For this review, take the finished solid that the model builds, in its own axes (mm). Face numbers are marked on the shaded views. A direction names the side the tool comes from. Coordinates: 2 decimals unless noted, no trailing zeros. Loops run counter-clockwise (first coordinate to the right, second up) from the corner with the lowest first, then second, coordinate; pieces in that order, holes last. Notation, with made-up numbers: (70, 89.5) - (82, 89.5) arc R9 ccw to (82, 105.5) - close; hole circle Ø1 at (53, -11.75). An arc over 180 degrees is marked (long way). One line per item, written item: value. Start each with the question number.
1. To check wall thickness, follow line 1 (X direction, y = -2.5, z = 9.75); line 2 (X direction, y = 2.75, z = 9.75); line 3 (Z direction, x = 62, y = 3.5). State the ranges of each line that lie inside material, in increasing order. Write a range as from..to.
2. Take a section at A-A, the plane z = 5.5. State the section outline as (x, y) points, and give its area (3 significant figures).
3. Insertion check: pin 1 (1 mm diameter, centred on y = -2.5, z = 2.5, fed in from -X); pin 2 (1.6 mm diameter, centred on x = 98, y = 1, fed in from -Z); pin 3 (1 mm diameter, centred on y = -3, z = 10.5, fed in from -X). Each pin has a flat end and moves straight along its axis. Give the tip position at first contact, or say it passes through.
4. For the marked faces 3 and 4, list the 3-axis set-ups (+Z, -Z, +X, -X, +Y, -Y) from which the entire face can be reached by the end or side of a thin tool; tool diameter is ignored.
5. The part is to be moulded in two halves that separate along X. For the marked faces 1 and 2, say which applies: released by +X, released by -X, zero draft, split by the parting line, or undercut.
6. Take a section at B-B, the plane x = 43.5. State the section outline as (y, z) points.
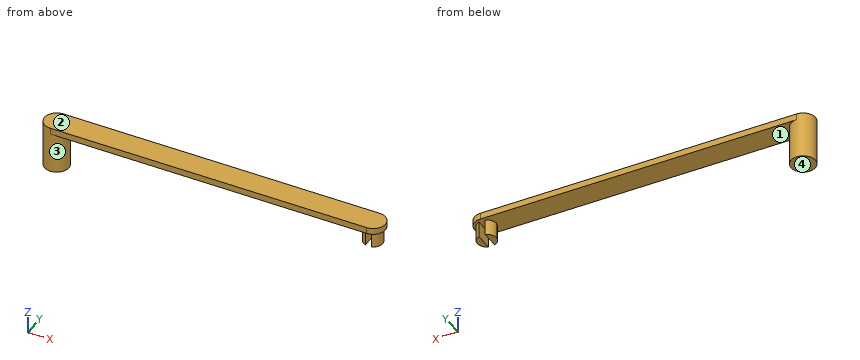
```python
from build123d import *

# Parameters (mm, degrees)
SKETCH1_R           = 3.85
BOSS_EXTRUDE1_DEPTH = 12.83
SKETCH2_R           = 3.85
BOSS_EXTRUDE3_DEPTH = 2
BOSS_EXTRUDE5_DEPTH = 5


with BuildPart() as part:
    # Sketch1 → Boss-Extrude1 (new body)
    with BuildSketch(Plane.XY):
        with Locations(Location((0, 0, 0), (0, 0, 180))):
            Circle(SKETCH1_R)
    extrude(amount=BOSS_EXTRUDE1_DEPTH)

    # Sketch2 → Boss-Extrude3 (add)
    with BuildSketch(Plane.XY.offset(12.83)):
        with Locations((100, 0)):
            Circle(SKETCH2_R)
        with BuildLine():
            Line((100, 3.85), (0, 3.85))
            ThreePointArc((0, 3.85), (2.722361108, 2.722361108), (3.85, 0))
            ThreePointArc((3.85, 0), (2.722361108, -2.722361108), (0, -3.85))
            Line((0, -3.85), (100, -3.85))
            ThreePointArc((100, -3.85), (96.15, 0), (100, 3.85))
        make_face()
        with BuildLine():
            ThreePointArc((3.85, 0), (2.722361108, 2.722361108), (0, 3.85))
            Line((0, 3.85), (0, -3.85))
            ThreePointArc((0, -3.85), (2.722361108, -2.722361108), (3.85, 0))
        make_face()
        with BuildLine():
            Line((0, -3.85), (0, 3.85))
            ThreePointArc((0, 3.85), (-3.85, 0), (0, -3.85))
        make_face()
    extrude(amount=BOSS_EXTRUDE3_DEPTH)

    # Sketch3 → Boss-Extrude5 (add)
    with BuildSketch(Plane(origin=(0, 0, 12.83), x_dir=(-1, 0, 0), z_dir=(0, 0, -1))):
        with BuildLine():
            Line((-101, -2.828427125), (-101, 2.828427125))
            ThreePointArc((-101, 2.828427125), (-103, 0), (-101, -2.828427125))
        make_face()
        with BuildLine():
            ThreePointArc((-97, 0), (-97.550510257, 1.732050808), (-99, 2.828427125))
            Line((-99, 2.828427125), (-99, -2.828427125))
            ThreePointArc((-99, -2.828427125), (-97.550510257, -1.732050808), (-97, 0))
        make_face()
    extrude(amount=BOSS_EXTRUDE5_DEPTH)


solid = part.part
```
Solutions:
1. line 1: -2.93..2.93, 98.34..99, 101..101.66
1. line 2: -2.69..2.69, 98.8..99, 101..101.2
1. line 3: 12.83..14.83
2. outline: circle Ø7.7 at (0, 0)
2. area: 46.6 mm2
3. pin 1: x = -3.29
3. pin 2: z = 7.83
3. pin 3: x = -2.93
4. face 3: -Z
4. face 4: -Z, +X, -X, +Y, -Y
5. face 1: undercut
5. face 2: zero draft
6. outline: (-3.85, 12.83) - (3.85, 12.83) - (3.85, 14.83) - (-3.85, 14.83) - close
